```python
from build123d import *

# Parameters (mm, degrees)
SKETCH1_W            = 279.4
SKETCH1_H            = 101.6
BOSS_EXTRUDE1_DEPTH  = 6.35
SKETCH2_R            = 13.97
BOSS_EXTRUDE3_DEPTH  = 5.55625
SKETCH9_R            = 11.1125
CUT_EXTRUDE4_DEPTH   = 4.445
CUT_EXTRUDE5_START   = -5.55625
SKETCH10_R           = 11.1125
CUT_EXTRUDE5_DEPTH   = 5.55625
SKETCH11_R           = 7.9375
CUT_EXTRUDE6_DEPTH   = 285.078633923
SKETCH12_R           = 6.35
CUT_EXTRUDE7_DEPTH   = 285.051619429
SKETCH22_W           = 63.5
SKETCH22_H           = 63.5
BOSS_EXTRUDE7_DEPTH  = 12.7
SKETCH25_W           = 50.8
SKETCH25_H           = 50.8
CUT_EXTRUDE11_DEPTH  = 15.875
SKETCH32_R           = 4.7625
CUT_EXTRUDE12_DEPTH  = 6.35
SKETCH38_W           = 46.99
SKETCH38_H           = 18.470251096
CUT_EXTRUDE13_DEPTH  = 6.35
SKETCH60_R           = 4.7625
CUT_EXTRUDE23_DEPTH  = 6.35
SKETCH64_R           = 4.7625
CUT_EXTRUDE24_DEPTH  = 285.264471927
SKETCH69_W           = 33.02
SKETCH69_H           = 6.35
BOSS_EXTRUDE10_DEPTH = 19.05
SKETCH70_R           = 4.7625
SKETCH70_R_2         = 2.54
CUT_EXTRUDE26_DEPTH  = 6.35


with BuildPart() as part:
    # Sketch1 → Boss-Extrude1 (new body)
    with BuildSketch(Plane(origin=(0, 0, 0), x_dir=(1, 0, 0), z_dir=(0, 1, 0))):
        with Locations((-139.7, 0)):
            Rectangle(SKETCH1_W, SKETCH1_H)
    extrude(amount=BOSS_EXTRUDE1_DEPTH)

    # Sketch2 → Boss-Extrude3 (add)
    with BuildSketch(Plane(origin=(0, 6.35, 0), x_dir=(1, 0, 0), z_dir=(0, 1, 0))):
        with Locations(Location((-258.510557857, 0, 0), (0, 0, 90))):
            Circle(SKETCH2_R)
    extrude(amount=BOSS_EXTRUDE3_DEPTH)

    # Sketch9 → Cut-Extrude4 (cut)
    with BuildSketch(Plane(origin=(0, 11.90625, 0), x_dir=(1, 0, 0), z_dir=(0, 1, 0))):
        with Locations(Location((-258.510557857, 0, 0), (0, 0, 270))):
            Circle(SKETCH9_R)
    extrude(amount=-CUT_EXTRUDE4_DEPTH, mode=Mode.SUBTRACT)

    # Sketch10 → Cut-Extrude5 (cut)
    with BuildSketch(Plane(origin=(0, 0, 0), x_dir=(-1, 0, 0), z_dir=(0, -1, 0)).offset(CUT_EXTRUDE5_START)):
        with Locations(Location((258.510557857, 0, 0), (0, 0, 270))):
            Circle(SKETCH10_R)
    extrude(amount=CUT_EXTRUDE5_DEPTH, mode=Mode.SUBTRACT)

    # Sketch11 → Cut-Extrude6 (cut, through all)
    with BuildSketch(Plane(origin=(0, 7.46125, 0), x_dir=(1, 0, 0), z_dir=(0, 1, 0))):
        with Locations(Location((-258.510557857, 0, 0), (0, 0, 270))):
            Circle(SKETCH11_R)
    extrude(amount=-CUT_EXTRUDE6_DEPTH, mode=Mode.SUBTRACT)

    # Sketch12 → Cut-Extrude7 (cut, through all)
    with BuildSketch(Plane(origin=(0, 6.35, 0), x_dir=(1, 0, 0), z_dir=(0, 1, 0))):
        with Locations(Location((-134.666203771, 0, 0), (0, 0, 270))):
            Circle(SKETCH12_R)
    extrude(amount=-CUT_EXTRUDE7_DEPTH, mode=Mode.SUBTRACT)

    # Sketch22 → Boss-Extrude7 (add)
    with BuildSketch(Plane(origin=(0, 6.35, 0), x_dir=(1, 0, 0), z_dir=(0, 1, 0))):
        with Locations((-134.666203771, 0)):
            Rectangle(SKETCH22_W, SKETCH22_H)
    extrude(amount=BOSS_EXTRUDE7_DEPTH)

    # Sketch25 → Cut-Extrude11 (cut)
    with BuildSketch(Plane(origin=(0, 19.05, 0), x_dir=(1, 0, 0), z_dir=(0, 1, 0))):
        with Locations((-134.666203771, 0)):
            Rectangle(SKETCH25_W, SKETCH25_H)
    extrude(amount=-CUT_EXTRUDE11_DEPTH, mode=Mode.SUBTRACT)

    # Sketch32 → Cut-Extrude12 (cut)
    with BuildSketch(Plane(origin=(0, 6.35, 0), x_dir=(1, 0, 0), z_dir=(0, 1, 0))):
        with Locations(Location((-67.44195898, -40.64, 0), (0, 0, 270))):
            Circle(SKETCH32_R)
        with Locations(Location((-81.41195898, -40.64, 0), (0, 0, 270))):
            Circle(SKETCH32_R)
        with Locations(Location((-67.44195898, 40.64, 0), (0, 0, 270))):
            Circle(SKETCH32_R)
        with Locations(Location((-81.41195898, 40.64, 0), (0, 0, 270))):
            Circle(SKETCH32_R)
    extrude(amount=-CUT_EXTRUDE12_DEPTH, mode=Mode.SUBTRACT)

    # Sketch38 → Cut-Extrude13 (cut)
    with BuildSketch(Plane(origin=(0, 6.35, 0), x_dir=(1, 0, 0), z_dir=(0, 1, 0))):
        with Locations((-23.495, -24.777709652)):
            Rectangle(SKETCH38_W, SKETCH38_H)
    extrude(amount=-CUT_EXTRUDE13_DEPTH, mode=Mode.SUBTRACT)

    # Sketch60 → Cut-Extrude23 (cut)
    with BuildSketch(Plane(origin=(0, 6.35, 0), x_dir=(1, 0, 0), z_dir=(0, 1, 0))):
        with Locations(Location((-231.7492444, 41.324145444, 0), (0, 0, 270))):
            Circle(SKETCH60_R)
        with Locations(Location((-231.7492444, -39.369341378, 0), (0, 0, 270))):
            Circle(SKETCH60_R)
        with Locations(Location((-173.509244294, -39.369341378, 0), (0, 0, 270))):
            Circle(SKETCH60_R)
        with Locations(Location((-173.509244294, 41.324145444, 0), (0, 0, 270))):
            Circle(SKETCH60_R)
    extrude(amount=-CUT_EXTRUDE23_DEPTH, mode=Mode.SUBTRACT)

    # Sketch64 → Cut-Extrude24 (cut, through all)
    with BuildSketch(Plane(origin=(0, 6.35, 0), x_dir=(1, 0, 0), z_dir=(0, 1, 0))):
        with Locations(Location((-145.334203771, -41.275, 0), (0, 0, 270))):
            Circle(SKETCH64_R)
        with Locations(Location((-123.998203771, -41.275, 0), (0, 0, 270))):
            Circle(SKETCH64_R)
    cut_extrude24 = extrude(amount=-CUT_EXTRUDE24_DEPTH, mode=Mode.SUBTRACT)

    # Mirror1: Cut-Extrude24 across plane
    add(cut_extrude24.mirror(Plane.XY), mode=Mode.SUBTRACT)

    # Sketch69 → Boss-Extrude10 (add)
    with BuildSketch(Plane.XY.offset(50.8)):
        with Locations((-70.465355554, 3.175)):
            Rectangle(SKETCH69_W, SKETCH69_H)
    boss_extrude10 = extrude(amount=BOSS_EXTRUDE10_DEPTH)

    # Sketch70 → Cut-Extrude26 (cut)
    with BuildSketch(Plane(origin=(0, 6.35, 0), x_dir=(1, 0, 0), z_dir=(0, 1, 0))):
        with Locations(Location((-76.815355554, -60.325, 0), (0, 0, 270))):
            Circle(SKETCH70_R)
        with Locations(Location((-64.115355554, -60.325, 0), (0, 0, 270))):
            Circle(SKETCH70_R_2)
    cut_extrude26 = extrude(amount=-CUT_EXTRUDE26_DEPTH, mode=Mode.SUBTRACT)

    # Mirror2: Boss-Extrude10, Cut-Extrude26 across plane
    add(boss_extrude10.mirror(Plane.XY))
    add(cut_extrude26.mirror(Plane.XY), mode=Mode.SUBTRACT)


solid = part.part
```
Verification items for the finished model (mm, model axes). A direction names the side the tool comes from. Coordinates: 2 decimals unless noted, no trailing zeros. Loops run counter-clockwise (first coordinate to the right, second up) from the corner with the lowest first, then second, coordinate; pieces in that order, holes last. Notation, with made-up numbers: (6, -18.75) -> (31, -18.75) arc R12 cw to (31, -11.75) -> close; hole circle Ø6 at (80, -5). An arc over 180 degrees is marked (long way). Answer in a Markdown table with one row per item. Add a question column.
1. Section check D-D, the plane z = 40.64. Enter the section's corners in (x, y), then the cut area to 3 significant figures.
2. Depth check by flat-ended pin: P1, Ø7.5, axis at x = -145.33, z = -41.28, coming from the +Y side; P2, Ø7, axis at x = -29, y = 4.5, coming from the -Z side; P3, Ø1.9, axis at x = -15.5, y = 2.5, coming from the +Z side; P4, Ø10, axis at x = -144, y = 15, coming from the -Z side. Enter the tip coordinate at first touch or a pass-through.
3. Material ranges on probe 1 along Z at (x, y) = (-159, 18.25); probe 2 along X at (y, z) = (16.5, -3.5); probe 3 along Z at (x, y) = (-42, 3.5), recorded low to high. Write a range as [from, to].
4. Section check A-A, the plane z = 0. Give the number of separate pieces and of enclosed holes in the cut face, then the cut area to 3 significant figures.
5. Section check C-C, the plane z = -40.64. Enter the section's corners in (x, y), then the cut area to 3 significant figures.
6. Access from +Z, -Z, +X, -X, +Y, -Y to the whole of each face (thin tool, end or side, straight path). Record for faces 4 (the face through (-135, 13, -31.75)), 5 (the face through (-24, 3, 34.013)), 6 (the face through (-261, 5.556, -8)).
7. Draft check along X on faces 1 (the face through (-135, 13, 31.75)), 2 (the face through (-53.955, 3, 60)), 3 (the face through (-109.266, 11, 0)). Enter one of: +X half, -X half, draft (parallel to the pull), parting line (faces both ways), or undercut.
8. Section check B-B, the plane x = -154. Enter the section's corners in (y, z) (3 decimals).
Derived:
| question | item | result |
|---|---|---|
| 1 | outline | (-279.4, 0) -> (-236.34, 0) -> (-236.34, 6.35) -> (-279.4, 6.35) -> close; (-227.16, 0) -> (-178.1, 0) -> (-178.1, 6.35) -> (-227.16, 6.35) -> close; (-168.92, 0) -> (-150.05, 0) -> (-150.05, 6.35) -> (-168.92, 6.35) -> close; (-140.61, 0) -> (-128.72, 0) -> (-128.72, 6.35) -> (-140.61, 6.35) -> close; (-119.28, 0) -> (-86.17, 0) -> (-86.17, 6.35) -> (-119.28, 6.35) -> close; (-76.65, 0) -> (-72.2, 0) -> (-72.2, 6.35) -> (-76.65, 6.35) -> close; (-62.68, 0) -> (0, 0) -> (0, 6.35) -> (-62.68, 6.35) -> close |
| 1 | area | 1,420 mm² |
| 2 | P1 | passes through |
| 2 | P2 | stops at z = -50.8 |
| 2 | P3 | stops at z = 50.8 |
| 2 | P4 | stops at z = -31.75 |
| 3 | probe 1 | z = [-31.75, -25.4], [25.4, 31.75] |
| 3 | probe 2 | x = [-166.42, -160.07], [-109.27, -102.92] |
| 3 | probe 3 | z = [-50.8, 15.54], [34.01, 50.8] |
| 4 | separate pieces | 3 |
| 4 | enclosed holes | 0 |
| 4 | area | 1,640 mm² |
| 5 | outline | (-279.4, 0) -> (-236.46, 0) -> (-236.46, 6.35) -> (-279.4, 6.35) -> close; (-227.04, 0) -> (-178.22, 0) -> (-178.22, 6.35) -> (-227.04, 6.35) -> close; (-168.8, 0) -> (-150.05, 0) -> (-150.05, 6.35) -> (-168.8, 6.35) -> close; (-140.61, 0) -> (-128.72, 0) -> (-128.72, 6.35) -> (-140.61, 6.35) -> close; (-119.28, 0) -> (-86.17, 0) -> (-86.17, 6.35) -> (-119.28, 6.35) -> close; (-76.65, 0) -> (-72.2, 0) -> (-72.2, 6.35) -> (-76.65, 6.35) -> close; (-62.68, 0) -> (0, 0) -> (0, 6.35) -> (-62.68, 6.35) -> close |
| 5 | area | 1,410 mm² |
| 6 | face 4 | -Z, +X, -X, +Y |
| 6 | face 5 | +X, +Y, -Y |
| 6 | face 6 | -Y |
| 7 | face 1 | draft |
| 7 | face 2 | +X half |
| 7 | face 3 | undercut |
| 8 | outline | (0, -50.8) -> (6.35, -50.8) -> (6.35, -31.75) -> (19.05, -31.75) -> (19.05, -25.4) -> (3.175, -25.4) -> (3.175, 25.4) -> (19.05, 25.4) -> (19.05, 31.75) -> (6.35, 31.75) -> (6.35, 50.8) -> (0, 50.8) -> close |
